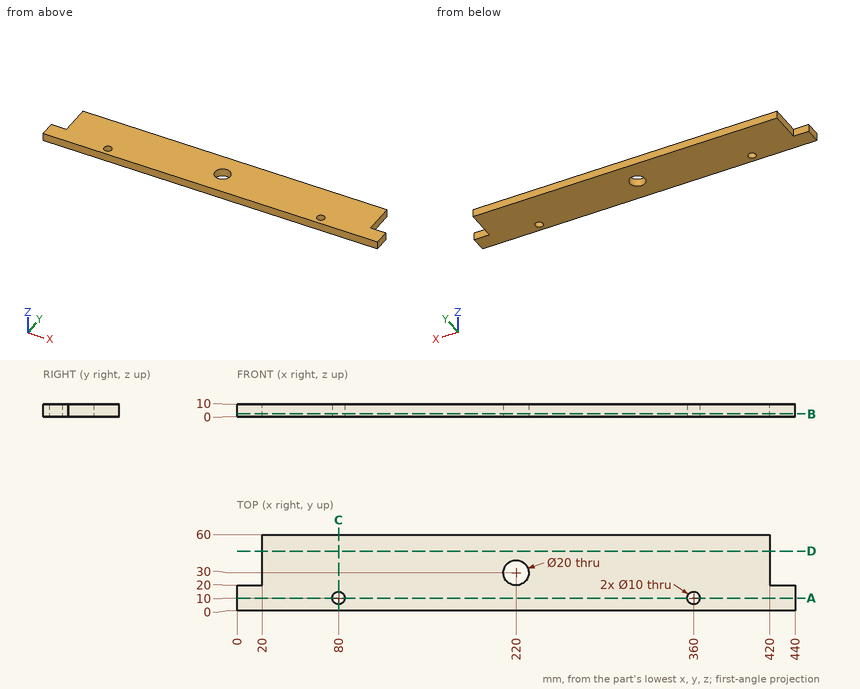
Verification items for this drawing (mm, ordinates from the low corner). Coordinates: 2 decimals unless noted, no trailing zeros. Loops run counter-clockwise (first coordinate to the right, second up) from the corner with the lowest first, then second, coordinate; pieces in that order, holes last. Notation, with made-up numbers: (-9, -16.75) - (23, -16.75) arc R20 cw to (23, 7.25) - close; hole circle Ø4 at (15, 10). An arc over 180 degrees is marked (long way). One line per item, written item: value. Start each with the question number.
(1) Cross-section at C-C on x = 80. Enter the section's corners in (y, z).
(2) Cross-section at A-A on y = 10. Enter the section's corners in (x, z).
(3) Material ranges on line 1 (X direction, y = 10, z = 3.75); line 2 (Y direction, x = 360, z = 4.5); line 3 (Y direction, x = 220, z = 5), recorded low to high. Write a range as [from, to].
(4) Depth check by flat-ended pin: P1, Ø5, axis at x = 428.5, z = 5.5, coming from the +Y side; P2, Ø3, axis at y = 48, z = 5, coming from the -X side; P3, Ø9, axis at x = 80, y = 10, coming from the +Z side. Enter the tip coordinate at first touch or a pass-through.
(5) Cross-section at D-D on y = 47. Enter the section's corners in (x, z), plus the area to 3 significant figures.
(6) Cross-section at B-B on z = 2.25. Enter the section's corners in (x, y), plus the area to 3 significant figures.
Results below:
1. outline: (0, 0) - (5, 0) - (5, 10) - (0, 10) - close; (15, 0) - (60, 0) - (60, 10) - (15, 10) - close
2. outline: (0, 0) - (75, 0) - (75, 10) - (0, 10) - close; (85, 0) - (355, 0) - (355, 10) - (85, 10) - close; (365, 0) - (440, 0) - (440, 10) - (365, 10) - close
3. line 1: x = [0, 75], [85, 355], [365, 440]
3. line 2: y = [0, 5], [15, 60]
3. line 3: y = [0, 20], [40, 60]
4. P1: stops at y = 20
4. P2: stops at x = 20
4. P3: passes through
5. outline: (20, 0) - (420, 0) - (420, 10) - (20, 10) - close
5. area: 4,000 mm2
6. outline: (0, 0) - (440, 0) - (440, 20) - (420, 20) - (420, 60) - (20, 60) - (20, 20) - (0, 20) - close; hole circle Ø10 at (80, 10); hole circle Ø20 at (220, 30); hole circle Ø10 at (360, 10)
6. area: 24,300 mm2
